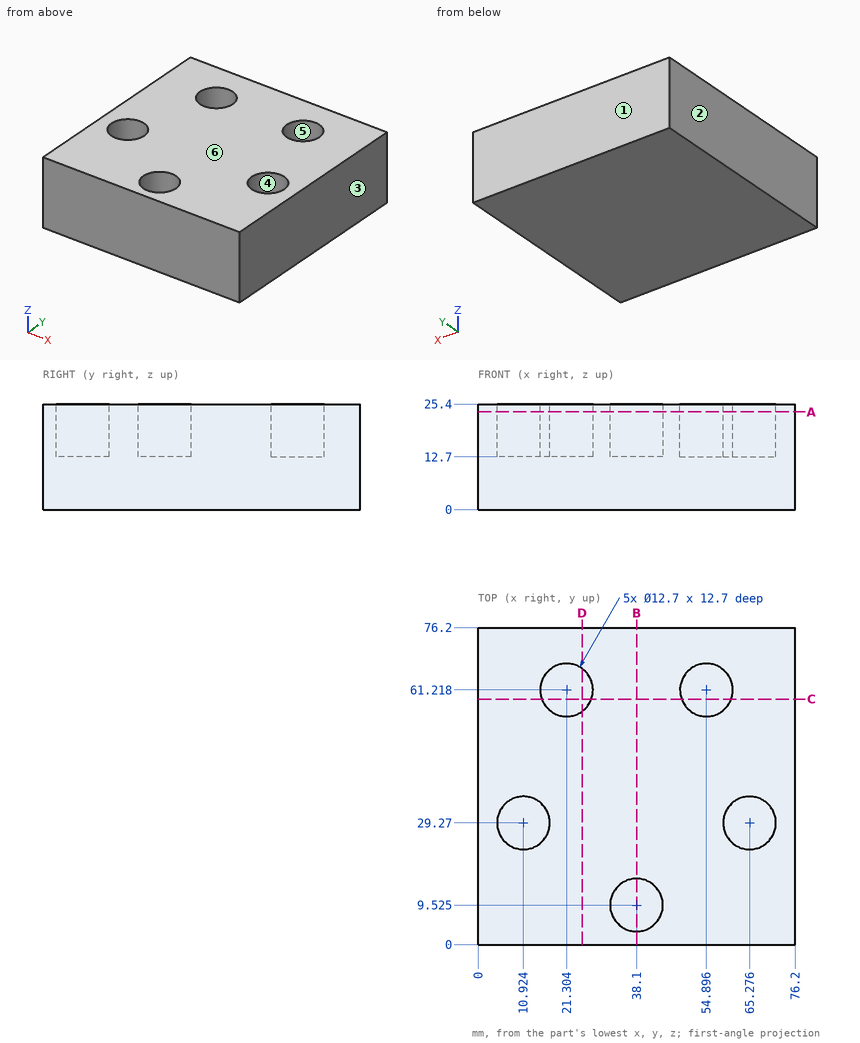
Print and shaded views of the part. All mm, measured from the part's lowest x, y and z. A direction names the side the tool comes from. Round coordinates to 2 decimals unless told otherwise and drop trailing zeros. Write each loop counter-clockwise with the first axis right and the second up, starting at its lowest first coordinate (ties: lowest second). Pieces come first, ordered by that corner, then holes. Notation, with made-up numbers: (20.25, 24.25) -> (44.25, 24.25) arc R32 ccw to (44.25, 53.25) -> close; hole circle Ø8 at (46.25, 50). An arc over 180 degrees is marked (long way). Return JSON: item names as keys, results as strings. Group by question number.
Q1. Saw through at C-C on y = 59. Write the cut outline in (x, z) (1 decimal), plus the area to 3 significant figures.
Q2. Saw through at A-A on z = 23.5. State how many separate pieces and enclosed holes the cut face has, plus the area to 3 significant figures.
Q3. Mould opens along X. For the marked faces 1, 2, 3 and 4 say: pulls with the +X half, pulls with the -X half, needs draft (parallel to the pull), parting line crosses it, or undercut.
Q4. Probe L1, parallel to X at y = 64.5, z = 17; L2, parallel to Y at x = 38.5, z = 20.5; L3, parallel to Z at x = 68, y = 31. List the from-to ranges inside material, lowest first. Write a range as [from, to].
Q5. Saw through at B-B on x = 38.1. Write the cut outline in (y, z) (1 decimal).
Q6. Pin check, flat tip, straight feed: pin 1 (6 mm diameter, centred on x = 20, y = 61.5, fed in from +Z). Stop position of the tip, or through.
Q7. Saw through at D-D on x = 25. Write the cut outline in (y, z).
Q8. Which spindle directions (+Z, -Z, +X, -X, +Y, -Y) get a long thin tool onto all of the face, cutting with end or side? Do the marked faces 5 and 6. Say none if no direction does.
Answer:
{
 "1": {"outline": "(0, 0) -> (76.2, 0) -> (76.2, 25.4) -> (60.8, 25.4) -> (60.8, 12.7) -> (48.9, 12.7) -> (48.9, 25.4) -> (27.3, 25.4) -> (27.3, 12.7) -> (15.4, 12.7) -> (15.4, 25.4) -> (0, 25.4) -> close", "area": "1,630 mm2"},
 "2": {"separate pieces": "1", "enclosed holes": "5", "area": "5,170 mm2"},
 "3": {"face 1": "needs draft", "face 2": "pulls with the -X half", "face 3": "pulls with the +X half", "face 4": "undercut"},
 "4": {"L1": "[0, 15.87], [26.74, 49.46], [60.33, 76.2]", "L2": "[0, 3.19], [15.86, 76.2]", "L3": "[0, 12.7]"},
 "5": {"outline": "(0, 0) -> (76.2, 0) -> (76.2, 25.4) -> (15.9, 25.4) -> (15.9, 12.7) -> (3.2, 12.7) -> (3.2, 25.4) -> (0, 25.4) -> close"},
 "6": {"pin 1": "z = 12.7"},
 "7": {"outline": "(0, 0) -> (76.2, 0) -> (76.2, 25.4) -> (66.38, 25.4) -> (66.38, 12.7) -> (56.05, 12.7) -> (56.05, 25.4) -> (0, 25.4) -> close"},
 "8": {"face 5": "+Z", "face 6": "+Z, +X, -X, +Y, -Y"}
}
